The model under review builds one solid part; all positions refer to its coordinate system, in mm. A direction names the side the tool comes from. Give positions to 0.01 mm unless a question says otherwise; leave off trailing zeros. Loops run counter-clockwise (first coordinate to the right, second up) from the corner with the lowest first, then second, coordinate; pieces in that order, holes last. Notation, with made-up numbers: M 71,48 L 91,48 A30 ccw 91,83 Z; hole C 87,89.25 d6. An arc over 180 degrees is marked long. Return JSON: item names as keys, results as strings. Group by question number.
```python
from build123d import *

# Parameters (mm, degrees)
SKETCH1_R           = 10
SKETCH1_R_2         = 1.25
SKETCH1_R_3         = 1.5
BOSS_EXTRUDE1_DEPTH = 2
SKETCH2_R           = 4.625
SKETCH2_R_2         = 3
BOSS_EXTRUDE2_DEPTH = 2.5


with BuildPart() as part:
    # Sketch1 → Boss-Extrude1 (new body)
    with BuildSketch(Plane(origin=(0, 0, 0), x_dir=(1, 0, 0), z_dir=(0, 1, 0))):
        Circle(SKETCH1_R)
        with Locations((0, 7)):
            Circle(SKETCH1_R_2, mode=Mode.SUBTRACT)
        Circle(SKETCH1_R_3, mode=Mode.SUBTRACT)
        with Locations((7, 0)):
            Circle(SKETCH1_R_2, mode=Mode.SUBTRACT)
        with Locations((0, -7)):
            Circle(SKETCH1_R_2, mode=Mode.SUBTRACT)
        with Locations((-7, 0)):
            Circle(SKETCH1_R_2, mode=Mode.SUBTRACT)
    extrude(amount=BOSS_EXTRUDE1_DEPTH)

    # Sketch2 → Boss-Extrude2 (add)
    with BuildSketch(Plane(origin=(0, 2, 0), x_dir=(1, 0, 0), z_dir=(0, 1, 0))):
        Circle(SKETCH2_R)
        Circle(SKETCH2_R_2, mode=Mode.SUBTRACT)
    extrude(amount=BOSS_EXTRUDE2_DEPTH)


solid = part.part
```
(1) Add section B-B (z = 0). Write out the cut boundary in (x, y) (3 decimals), and give its area (3 significant figures).
(2) For pin 1 (2 mm diameter, centred on x = 2.5, y = 2, fed in from +Z); pin 2 (1.8 mm diameter, centred on x = -1.5, z = -1, fed in from +Y), all flat-tipped, find the tip position at first contact; note any pin that passes through.
(3) Add section C-C (x = 7). Write out the cut boundary in (y, z), and give its area (3 significant figures).
(4) For probe 1 along Z at (x, y) = (0, 0.8); probe 2 along Y at (x, z) = (6.75, 3.25); probe 3 along X at (y, z) = (1.4, 7), list the stretches that pass through material, from the lowest coordinate up.
(5) Mouldability with a two-part tool opening along Z and no side actions: class faces 1 (the cylindrical face through (-3, 3, 0)), 2 (the flat face through (0, 0, 2)), 3 (the cylindrical face through (-1.003, 3.232, 4.515)) as released by +Z, released by -Z, zero draft, split by the parting line, or undercut.
(6) Add section D-D (z = -6.5). Write out the cut boundary in (x, y), and give its area (3 significant figures).
(7) For faces 4 (the cylindrical face through (-1.5, 0.99, -0.07)), 5 (the flat face through (2.1, 2, 4.3)), list the 3-axis set-ups (+Z, -Z, +X, -X, +Y, -Y) from which the entire face can be reached by the end or side of a thin tool; tool diameter is ignored.
(8) Add section A-A (x = 0). Write out the cut boundary in (y, z) (3 decimals), and give its area (3 significant figures).
Verdict:
{
 "1": {"outline": "M -10,0 L -8.25,0 L -8.25,2 L -10,2 Z; M -5.75,0 L -1.5,0 L -1.5,2 L -3,2 L -3,4.5 L -4.625,4.5 L -4.625,2 L -5.75,2 Z; M 1.5,0 L 5.75,0 L 5.75,2 L 4.625,2 L 4.625,4.5 L 3,4.5 L 3,2 L 1.5,2 Z; M 8.25,0 L 10,0 L 10,2 L 8.25,2 Z", "area": "32.1 mm²"},
 "2": {"pin 1": "stops at z = 9.89", "pin 2": "stops at y = 2"},
 "3": {"outline": "M 0,-7.14 L 2,-7.14 L 2,-1.25 L 0,-1.25 Z; M 0,1.25 L 2,1.25 L 2,7.14 L 0,7.14 Z", "area": "23.6 mm²"},
 "4": {"probe 1": "z = -10 to -8.25, -5.75 to -1.5, 1.5 to 5.75, 8.25 to 10", "probe 2": "y = 0 to 2", "probe 3": "x = -7.14 to -1.25, 1.25 to 7.14"},
 "5": {"face 1": "undercut", "face 2": "zero draft", "face 3": "split by the parting line"},
 "6": {"outline": "M -7.6,0 L -1.15,0 L -1.15,2 L -7.6,2 Z; M 1.15,0 L 7.6,0 L 7.6,2 L 1.15,2 Z", "area": "25.8 mm²"},
 "7": {"face 4": "+Y, -Y", "face 5": "+Y"},
 "8": {"outline": "M 0,-10 L 2,-10 L 2,-8.25 L 0,-8.25 Z; M 0,-5.75 L 2,-5.75 L 2,-4.625 L 4.5,-4.625 L 4.5,-3 L 2,-3 L 2,-1.5 L 0,-1.5 Z; M 0,1.5 L 2,1.5 L 2,3 L 4.5,3 L 4.5,4.625 L 2,4.625 L 2,5.75 L 0,5.75 Z; M 0,8.25 L 2,8.25 L 2,10 L 0,10 Z", "area": "32.1 mm²"}
}
